from build123d import *

# Parameters (mm, degrees)
BOSS_EXTRUDE1_DEPTH                           = 12
CBORE_FOR_M10_HEX_HEAD_CAP_SCREW1_D           = 11
CBORE_FOR_M10_HEX_HEAD_CAP_SCREW1_CBORE_D     = 21.475
CBORE_FOR_M10_HEX_HEAD_CAP_SCREW1_CBORE_DEPTH = 6.4
SKETCH4_R                                     = 17.5
SKETCH4_R_2                                   = 5
BOSS_EXTRUDE3_DEPTH                           = 24
SKETCH7_R                                     = 5
SKETCH7_R_2                                   = 17.5
BOSS_EXTRUDE4_DEPTH                           = 12
CUT_EXTRUDE2_START                            = -48
CUT_EXTRUDE2_OUTLINE_R                        = 5
CUT_EXTRUDE2_OUTLINE_R_2                      = 17.5
CUT_EXTRUDE2_DEPTH                            = 36


# Read off the part's stored shape, not the designer's step: Cut-Extrude2
with BuildPart() as part:
    # Sketch1 → Boss-Extrude1 (new body)
    with BuildSketch(Plane(origin=(0, 0, 0), x_dir=(1, 0, 0), z_dir=(0, 1, 0))):
        with BuildLine():
            Line((-60, -33.757736606), (60, -33.757736606))
            ThreePointArc((60, -33.757736606), (67.707641844, -28.846955004), (70, -20))
            Line((70, -20), (70, 20))
            ThreePointArc((70, 20), (67.707641844, 28.846955004), (60, 33.757736606))
            Line((60, 33.757736606), (-60, 33.757736606))
            ThreePointArc((-60, 33.757736606), (-67.707641844, 28.846955004), (-70, 20))
            Line((-70, 20), (-70, -20))
            ThreePointArc((-70, -20), (-67.707641844, -28.846955004), (-60, -33.757736606))
        make_face()
    extrude(amount=BOSS_EXTRUDE1_DEPTH)

    # CBORE for M10 Hex Head Cap Screw1 (through all)
    with Locations(Plane(origin=(-57.615806102, 12, -21.511565447), x_dir=(0, 0, 1), z_dir=(0, 1, 0))):
        with Locations((0, 0), (43.023130894, 0), (43.023130894, 115.231612204), (0, 115.231612204)):
            CounterBoreHole(CBORE_FOR_M10_HEX_HEAD_CAP_SCREW1_D / 2, CBORE_FOR_M10_HEX_HEAD_CAP_SCREW1_CBORE_D / 2, CBORE_FOR_M10_HEX_HEAD_CAP_SCREW1_CBORE_DEPTH)

    # Sketch4 → Boss-Extrude3 (add)
    # profile 1 of 11: a face of its own
    with BuildSketch(Plane(origin=(0, 12, 0), x_dir=(1, 0, 0), z_dir=(0, 1, 0))):
        with BuildLine():
            Line((-7, 24), (-37.5, 24))
            ThreePointArc((-37.5, 24), (-41.035533906, 22.535533906), (-42.5, 19))
            Line((-42.5, 19), (-42.5, 1.2e-07))
            ThreePointArc((-42.5, 1.2e-07), (-41.048504112, 5.188745268), (-37.115384615, 8.871201996))
            Line((-37.115384615, 8.871201996), (-11.538461538, 22.17800499))
            ThreePointArc((-11.538461538, 22.17800499), (-9.31389046, 23.200246647), (-7, 24))
        make_face()
    # profile 2 of 11: a face of its own
    with BuildSketch(Plane(origin=(0, 12, 0), x_dir=(1, 0, 0), z_dir=(0, 1, 0))):
        with BuildLine():
            ThreePointArc((-37.115384615, -8.871201996), (-41.048504174, -5.188745165), (-42.5, 1.2e-07))
            Line((-42.5, 1.2e-07), (-42.5, -19))
            ThreePointArc((-42.5, -19), (-41.035533906, -22.535533906), (-37.5, -24))
            Line((-37.5, -24), (-7, -24))
            ThreePointArc((-7, -24), (-9.31389046, -23.200246647), (-11.538461538, -22.17800499))
            Line((-11.538461538, -22.17800499), (-37.115384615, -8.871201996))
        make_face()
    # profile 3 of 11: a face of its own
    with BuildSketch(Plane(origin=(0, 12, 0), x_dir=(1, 0, 0), z_dir=(0, 1, 0))):
        with BuildLine():
            Line((42.5, -19), (42.5, 1.1e-07))
            ThreePointArc((42.5, 1.1e-07), (41.048504171, -5.18874517), (37.115384615, -8.871201996))
            Line((37.115384615, -8.871201996), (11.538461538, -22.17800499))
            ThreePointArc((11.538461538, -22.17800499), (9.31389046, -23.200246647), (7, -24))
            Line((7, -24), (37.5, -24))
            ThreePointArc((37.5, -24), (41.035533906, -22.535533906), (42.5, -19))
        make_face()
    # profile 4 of 11: a face of its own
    with BuildSketch(Plane(origin=(0, 12, 0), x_dir=(1, 0, 0), z_dir=(0, 1, 0))):
        with BuildLine():
            Line((37.5, 24), (7, 24))
            ThreePointArc((7, 24), (9.31389046, 23.200246647), (11.538461538, 22.17800499))
            Line((11.538461538, 22.17800499), (37.115384615, 8.871201996))
            ThreePointArc((37.115384615, 8.871201996), (41.048504114, 5.188745264), (42.5, 1.1e-07))
            Line((42.5, 1.1e-07), (42.5, 19))
            ThreePointArc((42.5, 19), (41.035533906, 22.535533906), (37.5, 24))
        make_face()
    # profile 5 of 11: a face of its own
    with BuildSketch(Plane(origin=(0, 12, 0), x_dir=(1, 0, 0), z_dir=(0, 1, 0))):
        with BuildLine():
            Line((7, 24), (-7, 24))
            ThreePointArc((-7, 24), (-9.31389046, 23.200246647), (-11.538461538, 22.17800499))
            ThreePointArc((-11.538461538, 22.17800499), (-25, 0), (-11.538461538, -22.17800499))
            ThreePointArc((-11.538461538, -22.17800499), (-9.31389046, -23.200246647), (-7, -24))
            Line((-7, -24), (7, -24))
            ThreePointArc((7, -24), (9.31389046, -23.200246647), (11.538461538, -22.17800499))
            ThreePointArc((11.538461538, -22.17800499), (21.371260357, -12.971863042), (25, 0))
            ThreePointArc((25, 0), (21.371260357, 12.971863042), (11.538461538, 22.17800499))
            ThreePointArc((11.538461538, 22.17800499), (9.31389046, 23.200246647), (7, 24))
        make_face()
        with Locations(Location((0, 0, 0), (0, 0, 270))):
            Circle(SKETCH4_R, mode=Mode.SUBTRACT)
    # profile 6 of 11: a face of its own
    with BuildSketch(Plane(origin=(0, 12, 0), x_dir=(1, 0, 0), z_dir=(0, 1, 0))):
        with BuildLine():
            ThreePointArc((7, 24), (0, 25), (-7, 24))
            Line((-7, 24), (7, 24))
        make_face()
    # profile 7 of 11: a face of its own
    with BuildSketch(Plane(origin=(0, 12, 0), x_dir=(1, 0, 0), z_dir=(0, 1, 0))):
        with BuildLine():
            ThreePointArc((-11.538461538, -22.17800499), (-25, 0), (-11.538461538, 22.17800499))
            Line((-11.538461538, 22.17800499), (-37.115384615, 8.871201996))
            ThreePointArc((-37.115384615, 8.871201996), (-41.048504112, 5.188745268), (-42.5, 1.2e-07))
            ThreePointArc((-42.5, 1.2e-07), (-41.048504174, -5.188745165), (-37.115384615, -8.871201996))
            Line((-37.115384615, -8.871201996), (-11.538461538, -22.17800499))
        make_face()
        with Locations((-32.5, 0)):
            Circle(SKETCH4_R_2, mode=Mode.SUBTRACT)
    # profile 8 of 11: a face of its own
    with BuildSketch(Plane(origin=(0, 12, 0), x_dir=(1, 0, 0), z_dir=(0, 1, 0))):
        with BuildLine():
            Line((37.115384615, 8.871201996), (11.538461538, 22.17800499))
            ThreePointArc((11.538461538, 22.17800499), (21.371260357, 12.971863042), (25, 0))
            ThreePointArc((25, 0), (21.371260357, -12.971863042), (11.538461538, -22.17800499))
            Line((11.538461538, -22.17800499), (37.115384615, -8.871201996))
            ThreePointArc((37.115384615, -8.871201996), (41.048504171, -5.18874517), (42.5, 1.1e-07))
            ThreePointArc((42.5, 1.1e-07), (41.048504114, 5.188745264), (37.115384615, 8.871201996))
        make_face()
        with Locations((32.5, 0)):
            Circle(SKETCH4_R_2, mode=Mode.SUBTRACT)
    # profile 9 of 11: a face of its own
    with BuildSketch(Plane(origin=(0, 12, 0), x_dir=(1, 0, 0), z_dir=(0, 1, 0))):
        with Locations((32.5, 0)):
            Circle(SKETCH4_R_2)
    # profile 10 of 11: a face of its own
    with BuildSketch(Plane(origin=(0, 12, 0), x_dir=(1, 0, 0), z_dir=(0, 1, 0))):
        with Locations((-32.5, 0)):
            Circle(SKETCH4_R_2)
    # profile 11 of 11: a face of its own
    with BuildSketch(Plane(origin=(0, 12, 0), x_dir=(1, 0, 0), z_dir=(0, 1, 0))):
        with BuildLine():
            Line((7, -24), (-7, -24))
            ThreePointArc((-7, -24), (0, -25), (7, -24))
        make_face()
    extrude(amount=BOSS_EXTRUDE3_DEPTH)

    # Sketch7 → Boss-Extrude4 (add)
    # profile 1 of 3: a face of its own
    with BuildSketch(Plane(origin=(0, 36, 0), x_dir=(1, 0, 0), z_dir=(0, 1, 0))):
        with BuildLine():
            Line((-37.115384615, -8.871201996), (-11.538461538, -22.17800499))
            ThreePointArc((-11.538461538, -22.17800499), (-25, 0), (-11.538461538, 22.17800499))
            Line((-11.538461538, 22.17800499), (-37.115384615, 8.871201996))
            ThreePointArc((-37.115384615, 8.871201996), (-41.04850415, 5.188745205), (-42.5, -2.7e-08))
            ThreePointArc((-42.5, -2.7e-08), (-41.048504136, -5.188745228), (-37.115384615, -8.871201996))
        make_face()
        with Locations(Location((-32.5, 0, 0), (0, 0, 270))):
            Circle(SKETCH7_R, mode=Mode.SUBTRACT)
    # profile 2 of 3: a face of its own
    with BuildSketch(Plane(origin=(0, 36, 0), x_dir=(1, 0, 0), z_dir=(0, 1, 0))):
        with BuildLine():
            ThreePointArc((37.115384615, -8.871201996), (41.048504154, -5.188745198), (42.5, 4.3e-08))
            ThreePointArc((42.5, 4.3e-08), (41.048504131, 5.188745235), (37.115384615, 8.871201996))
            Line((37.115384615, 8.871201996), (11.538461538, 22.17800499))
            ThreePointArc((11.538461538, 22.17800499), (21.371260357, 12.971863042), (25, 0))
            ThreePointArc((25, 0), (21.371260357, -12.971863042), (11.538461538, -22.17800499))
            Line((11.538461538, -22.17800499), (37.115384615, -8.871201996))
        make_face()
        with Locations(Location((32.5, 0, 0), (0, 0, 270))):
            Circle(SKETCH7_R, mode=Mode.SUBTRACT)
    # profile 3 of 3: a face of its own
    with BuildSketch(Plane(origin=(0, 36, 0), x_dir=(1, 0, 0), z_dir=(0, 1, 0))):
        with BuildLine():
            ThreePointArc((-7, -24), (0, -25), (7, -24))
            ThreePointArc((7, -24), (9.31389046, -23.200246647), (11.538461538, -22.17800499))
            ThreePointArc((11.538461538, -22.17800499), (21.371260357, -12.971863042), (25, 0))
            ThreePointArc((25, 0), (21.371260357, 12.971863042), (11.538461538, 22.17800499))
            ThreePointArc((11.538461538, 22.17800499), (9.31389046, 23.200246647), (7, 24))
            ThreePointArc((7, 24), (0, 25), (-7, 24))
            ThreePointArc((-7, 24), (-9.31389046, 23.200246647), (-11.538461538, 22.17800499))
            ThreePointArc((-11.538461538, 22.17800499), (-25, 0), (-11.538461538, -22.17800499))
            ThreePointArc((-11.538461538, -22.17800499), (-9.31389046, -23.200246647), (-7, -24))
        make_face()
        with Locations(Location((0, 0, 0), (0, 0, 270))):
            Circle(SKETCH7_R_2, mode=Mode.SUBTRACT)
    extrude(amount=BOSS_EXTRUDE4_DEPTH)

    # Cut-Extrude2 outline → Cut-Extrude2 (cut)
    with BuildSketch(Plane(origin=(0, 48, 0), x_dir=(1, 0, 0), z_dir=(0, 1, 0)).offset(CUT_EXTRUDE2_START)):
        with Locations((-32.5, 0)):
            Circle(CUT_EXTRUDE2_OUTLINE_R)
        with Locations((32.5, 0)):
            Circle(CUT_EXTRUDE2_OUTLINE_R)
        Circle(CUT_EXTRUDE2_OUTLINE_R_2)
    extrude(amount=CUT_EXTRUDE2_DEPTH, mode=Mode.SUBTRACT)


solid = part.part
Model file for the job. Use its own axes, mm. A direction names the side the tool comes from. Round coordinates to 2 decimals unless told otherwise and drop trailing zeros. Order: outer loops, then holes, each group sorted by start corner. A loop starts at its lowest first (then second) coordinate and runs counter-clockwise, first axis right, second up. Notation, with made-up numbers: M 54.5,-18.75 L 59.5,-18.75 A33 cw 59.5,13.25 Z; hole C 67.25,48 d2. An arc over 180 degrees is marked long. Write each question's results on one line, items separated by ' | '. Start each with the question number.
(1) Which spindle directions (+Z, -Z, +X, -X, +Y, -Y) get a long thin tool onto all of the face, cutting with end or side? Do faces 1 (the face through (-41.07, 23.83, 22.5)), 2 (the face through (41, 23.83, 22.57)), 3 (the face through (68.26, 8.84, 20.11)), 4 (the face through (-22, 24, -24)), 5 (the face through (22, 24, -24)). Say none if no direction does.
(2) Two-plate mould, pull along X, no slides. Class faces 6 (the face through (-1, 12, 30)), 7 (the face through (67.784, 5.916, -28.741)), 8 (the face through (-24.148, 41.916, -15.618)), 9 (the face through (-35.59, 23.66, 3.93)): pulls with the +X half, pulls with the -X half, needs draft (parallel to the pull), parting line crosses it, or undercut.
(3) Probe probe 1 along X at (y, z) = (23, 0); probe 2 along X at (y, z) = (23, 3.5); probe 3 along Y at (x, z) = (-37.5, 30.5). List the from-to ranges inside material, lowest first. Write a range as from..to.
(4) Saw through at B-B, the plane y = 17.5. Give the cut face in (x, z).
(5) Saw through at C-C, the plane z = 3. Give the cut face in (x, y), then the cut area to 3 significant figures.
(6) Saw through at D-D, the plane y = 38. Give the cut face in (x, z), then the cut area to 3 significant figures.
(7) Drop flat-ended pins along their axis: pin 1 (6 mm diameter, centred on x = 32.5, z = 0, fed in from -Y); pin 2 (10 mm diameter, centred on y = 7, z = -13.5, fed in from +X); pin 3 (12 mm diameter, centred on x = 17, y = 25.5, fed in from +Z); pin 4 (23.5 mm diameter, centred on x = 53, z = 25.5, fed in from +Y). Give the stop position or say it passes through.
(8) Saw through at A-A, the plane x = 0. Give the cut face in (y, z), then the cut area to 3 significant figures.
Established:
1) face 1: +Z, -X, +Y | face 2: +Z, +X, +Y | face 3: +Y | face 4: -Z, -X, +Y | face 5: -Z, +X, +Y
2) face 6: needs draft | face 7: pulls with the +X half | face 8: pulls with the -X half | face 9: undercut
3) probe 1: x = -42.5..-37.5, -27.5..-17.5, 17.5..27.5, 37.5..42.5 | probe 2: x = -42.5..-36.07, -28.93..-17.15, 17.15..28.93, 36.07..42.5 | probe 3: y = 0..12
4) outline: M -42.5,-19 A5 ccw -37.5,-24 L -7,-24 A25 ccw 7,-24 L 37.5,-24 A5 ccw 42.5,-19 L 42.5,19 A5 ccw 37.5,24 L 7,24 A25 ccw -7,24 L -37.5,24 A5 ccw -42.5,19 Z; hole C -32.5,0 d10; hole C 0,0 d35; hole C 32.5,0 d10
5) outline: M -70,0 L -36.5,0 L -36.5,48 L -42.04,48 L -42.04,36 L -42.5,36 L -42.5,12 L -70,12 Z; M -28.5,0 L -17.24,0 L -17.24,48 L -28.5,48 Z; M 17.24,0 L 28.5,0 L 28.5,48 L 17.24,48 Z; M 36.5,0 L 70,0 L 70,12 L 42.5,12 L 42.5,36 L 42.04,36 L 42.04,48 L 36.5,48 Z | area: 2,310 mm^2
6) outline: M -37.12,-8.87 L -11.54,-22.18 A25 ccw 11.54,-22.18 L 37.12,-8.87 A10 ccw 37.12,8.87 L 11.54,22.18 A25 ccw -11.54,22.18 L -37.12,8.87 A10 ccw Z; hole C -32.5,0 d10; hole C 0,0 d35; hole C 32.5,0 d10 | area: 1,720 mm^2
7) pin 1: passes through | pin 2: stops at x = 70 | pin 3: stops at z = 24 | pin 4: stops at y = 12
8) outline: M 0,-33.76 L 12,-33.76 L 12,-25 L 48,-25 L 48,-17.5 L 0,-17.5 Z; M 0,17.5 L 48,17.5 L 48,25 L 12,25 L 12,33.76 L 0,33.76 Z | area: 930 mm^2
